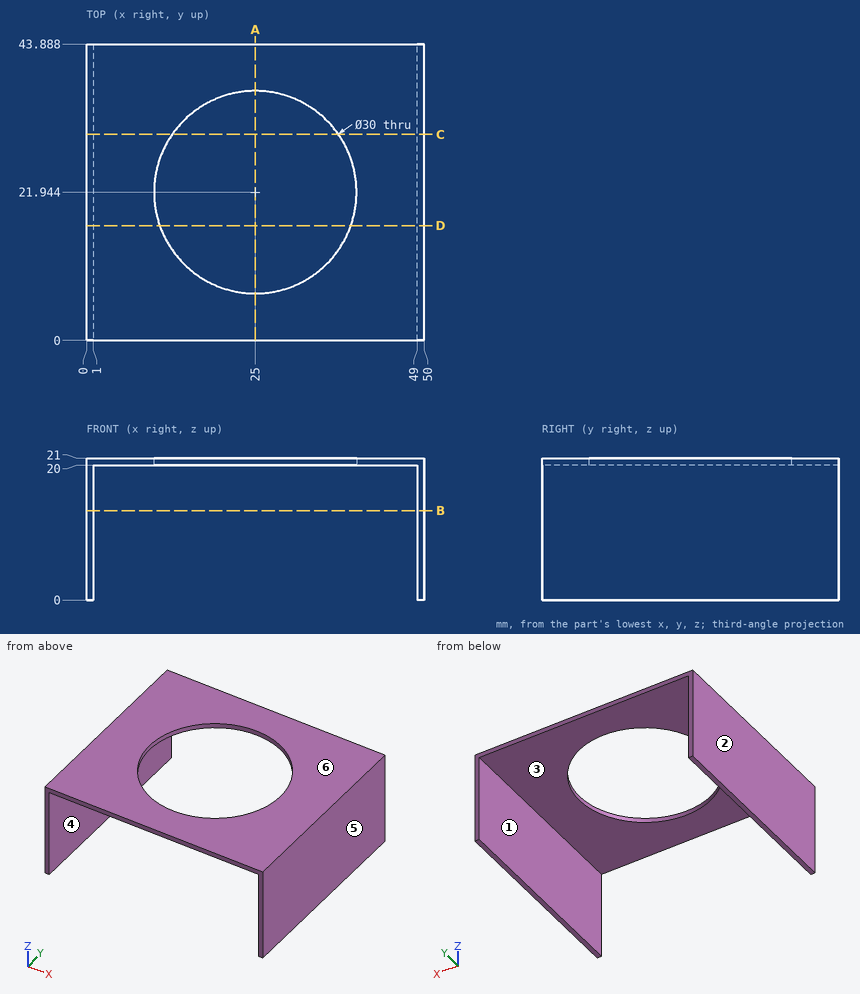
Verification items for this drawing (mm, ordinates from the low corner). A direction names the side the tool comes from. Round coordinates to 2 decimals unless told otherwise and drop trailing zeros. Loops run counter-clockwise (first coordinate to the right, second up) from the corner with the lowest first, then second, coordinate; pieces in that order, holes last. Notation, with made-up numbers: (38, -27.75) - (77, -27.75) arc R17 cw to (77, 0.25) - close; hole circle Ø5 at (78, -27). An arc over 180 degrees is marked (long way). Write item = value, one per line.
Q1. Material ranges on L1, parallel to X at y = 19.5, z = 14; L2, parallel to Y at x = 25, z = 20.5; L3, parallel to Z at x = 47.5, y = 13.5, recorded low to high.
Here are the results:
L1 = 0 to 1, 49 to 50
L2 = 0 to 6.94, 36.94 to 43.89
L3 = 20 to 21
Q2. Depth check by flat-ended pin: pin 1 (12 mm diameter, centred on x = 32, y = 10, fed in from +Z); pin 2 (12 mm diameter, centred on x = 13, y = 38.5, fed in from -Z). Enter the tip coordinate at first touch or a pass-through.
Here are the results:
pin_1 = 21
pin_2 = 20
Q3. Mould release check, pull along X, two halves, no side actions. Record for the marked faces 3, 4, 5 and 6: +X half, -X half, draft (parallel to the pull), parting line (faces both ways), or undercut.
Here are the results:
face_3 = undercut
face_4 = undercut
face_5 = +X half
face_6 = draft
Q4. Sectioned sample at A-A on x = 25. Record the boundary of the cut face in (y, z), plus the area to 3 significant figures.
Here are the results:
outline = (0, 20) - (6.94, 20) - (6.94, 21) - (0, 21) - close; (36.94, 20) - (43.89, 20) - (43.89, 21) - (36.94, 21) - close
area = 13.9 mm^2
Q5. Tool access check on the marked faces 1 and 2. Record the directions out of +Z, -Z, +X, -X, +Y, -Y that give a thin tool (end or side, any length) a straight path to the whole face; none if there is none.
Here are the results:
face_1 = -Z, +Y, -Y
face_2 = +Z, -Z, -X, +Y, -Y
Q6. Sectioned sample at B-B on z = 13.25. Record the boundary of the cut face in (x, y).
Here are the results:
outline = (0, 0) - (1, 0) - (1, 43.89) - (0, 43.89) - close; (49, 0) - (50, 0) - (50, 43.89) - (49, 43.89) - close
Q7. Sectioned sample at C-C on y = 30.5. Record the boundary of the cut face in (x, z).
Here are the results:
outline = (0, 0) - (1, 0) - (1, 20) - (12.68, 20) - (12.68, 21) - (0, 21) - close; (37.32, 20) - (49, 20) - (49, 0) - (50, 0) - (50, 21) - (37.32, 21) - close
Q8. Sectioned sample at D-D on y = 17. Record the boundary of the cut face in (x, z).
Here are the results:
outline = (0, 0) - (1, 0) - (1, 20) - (10.84, 20) - (10.84, 21) - (0, 21) - close; (39.16, 20) - (49, 20) - (49, 0) - (50, 0) - (50, 21) - (39.16, 21) - close
